from build123d import *

# Parameters (mm, degrees)
SKETCH2_R               = 73.3171
BOSS_EXTRUDE1_DEPTH     = 3.175
F_1_4_CLEARANCE_HOLE1_D = 6.7564
CUT_EXTRUDE1_START      = -4.175
CUT_EXTRUDE1_DEPTH      = 5.175
FILLET1_R               = 12.7
FILLET2_R               = 1.5875
FILLET1_OF_MIRROR1_R    = 12.7
FILLET2_OF_MIRROR1_R    = 1.5875


with BuildPart() as part:
    # Sketch2 → Boss-Extrude1 (new body)
    with BuildSketch(Plane(origin=(0, 0, 0), x_dir=(1, 0, 0), z_dir=(0, 1, 0))):
        Circle(SKETCH2_R)
    extrude(amount=BOSS_EXTRUDE1_DEPTH)

    # 1/4 Clearance Hole1 (through all)
    with Locations(Plane(origin=(0, 3.175, 0), x_dir=(1, 0, 0), z_dir=(0, 1, 0))):
        with Locations((-60.325, 0), (60.325, 0)):
            Hole(F_1_4_CLEARANCE_HOLE1_D / 2)

    # Sketch5 → Cut-Extrude1 (cut)
    with BuildSketch(Plane(origin=(0, 3.175, 0), x_dir=(1, 0, 0), z_dir=(0, 1, 0)).offset(CUT_EXTRUDE1_START)):
        Polygon((0, 63.2), (-15.802954744, 63.2), (-37.8, 50.5), (0, 50.5), align=None)
        Polygon((15.802954744, 63.2), (0, 63.2), (0, 50.5), (37.8, 50.5), align=None)
    cut_extrude1 = extrude(amount=CUT_EXTRUDE1_DEPTH, mode=Mode.SUBTRACT)

    # Fillet1
    fillet1_edges = [part.edges().sort_by_distance(p)[0] for p in [
        (-15.802954744, 1.5875, -63.2),
        (15.802954744, 1.5875, -63.2),
    ]]
    fillet(fillet1_edges, radius=FILLET1_R)

    # Fillet2
    fillet2_edges = [part.edges().sort_by_distance(p)[0] for p in [
        (-37.8, 1.5875, -50.5),
        (37.8, 1.5875, -50.5),
    ]]
    fillet(fillet2_edges, radius=FILLET2_R)

    # Mirror1: Cut-Extrude1 across plane
    add(cut_extrude1.mirror(Plane.XY), mode=Mode.SUBTRACT)

    # Fillet1 of Mirror1
    fillet1_of_mirror1_edges = [part.edges().sort_by_distance(p)[0] for p in [
        (-15.802954744, 1.5875, 63.2),
        (15.802954744, 1.5875, 63.2),
    ]]
    fillet(fillet1_of_mirror1_edges, radius=FILLET1_OF_MIRROR1_R)

    # Fillet2 of Mirror1
    fillet2_of_mirror1_edges = [part.edges().sort_by_distance(p)[0] for p in [
        (-37.8, 1.5875, 50.5),
        (37.8, 1.5875, 50.5),
    ]]
    fillet(fillet2_of_mirror1_edges, radius=FILLET2_OF_MIRROR1_R)


solid = part.part
CAD build for the part. Positions are in the model's coordinates, mm. A direction names the side the tool comes from. Give positions to 0.01 mm unless a question says otherwise; leave off trailing zeros. Write each loop counter-clockwise with the first axis right and the second up, starting at its lowest first coordinate (ties: lowest second). Pieces come first, ordered by that corner, then holes. Notation, with made-up numbers: M 56,-17.75 L 102,-17.75 A11 ccw 102,0.25 Z; hole C 8.5,75 d4. An arc over 180 degrees is marked long. Put each result on its own line as item: value. Start each with the question number.
(1) Band-saw the part on B-B, the plane z = 0. Write the cut outline in (x, y) (3 decimals), and give its area (3 significant figures).
(2) Which spindle directions (+Z, -Z, +X, -X, +Y, -Y) get a long thin tool onto all of the face, cutting with end or side? Do faces 1 (the face through (-25.61, 1.57, -57.54)), 2 (the face through (-1, 0, -1)). Say none if no direction does.
(3) Mould opens along Z. For faces 3 (the face through (-1, 3.175, -1)), 4 (the face through (0, 2, -50.5)), 5 (the face through (33.831, 1.565, 65.045)), 6 (the face through (25.807, 1.565, -57.424)) say: +Z half, -Z half, draft (parallel to the pull), parting line (faces both ways), or undercut.
(4) Band-saw the part on C-C, the plane y = 2.2. Give the number of separate pieces and of enclosed holes in the cut face, and give its area (3 significant figures).
(5) Flat gauge pins, fed straight in: pin 1 Ø9 at (x, z) = (60.325, 0) entering from -Y; pin 2 Ø1 at (x, y) = (-8, 2) entering from -Z; pin 3 Ø1 at (x, y) = (-15, 2) entering from +Z; pin 4 Ø4 at (x, z) = (-60.325, 0) entering from +Y. Where does each tip first touch, or does it go through?
(6) Band-saw the part on A-A, the plane x = 0. Write the cut outline in (y, z) (3 decimals), and give its area (3 significant figures).
(7) Band-saw the part on D-D, the plane x = 60. Write the cut outline in (y, z) (3 decimals).
(8) Probe L1, parallel to Z at x = 9.5, y = 0.85; L2, parallel to Z at x = 31, y = 1.4; L3, parallel to Z at x = -67, y = 0.2. List the from-to ranges inside material, lowest first.
Response values:
1. outline: M -73.317,0 L -63.703,0 L -63.703,3.175 L -73.317,3.175 Z; M -56.947,0 L 56.947,0 L 56.947,3.175 L -56.947,3.175 Z; M 63.703,0 L 73.317,0 L 73.317,3.175 L 63.703,3.175 Z
1. area: 423 mm2
2. face 1: +Y, -Y
2. face 2: +Z, -Z, +X, -X, -Y
3. face 3: draft
3. face 4: undercut
3. face 5: parting line
3. face 6: undercut
4. separate pieces: 1
4. enclosed holes: 4
4. area: 15,500 mm2
5. pin 1: stops at y = 0
5. pin 2: stops at z = -72.93
5. pin 3: stops at z = 71.87
5. pin 4: passes through
6. outline: M 0,-73.317 L 3.175,-73.317 L 3.175,-63.2 L 0,-63.2 Z; M 0,-50.5 L 3.175,-50.5 L 3.175,50.5 L 0,50.5 Z; M 0,63.2 L 3.175,63.2 L 3.175,73.317 L 0,73.317 Z
6. area: 385 mm2
7. outline: M 0,-42.135 L 3.175,-42.135 L 3.175,-3.363 L 0,-3.363 Z; M 0,3.363 L 3.175,3.363 L 3.175,42.135 L 0,42.135 Z
8. L1: z = -72.7 to -63.2, -50.5 to 50.5, 63.2 to 72.7
8. L2: z = -66.44 to -54.43, -50.5 to 50.5, 54.43 to 66.44
8. L3: z = -29.77 to 29.77
